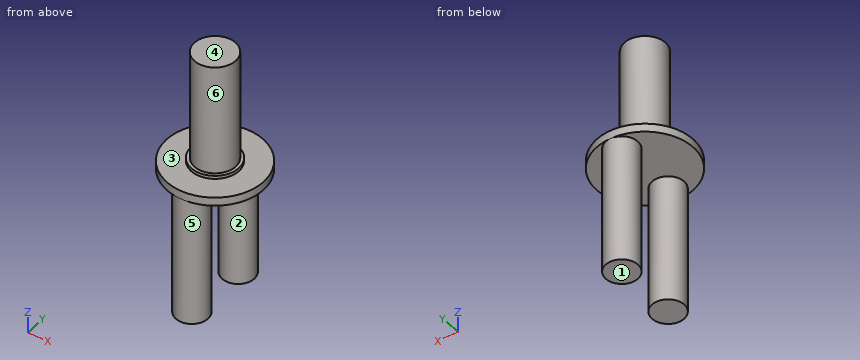
```python
from build123d import *

# Parameters (mm, degrees)
SKETCH1_R             = 1.5875
BOSS_EXTRUDE1_DEPTH   = 12.7
BOSS_EXTRUDE1_2_DEPTH = 12.7
SKETCH2_R             = 2.032
BOSS_EXTRUDE2_DEPTH   = 12.065
SKETCH3_R             = 4.7625
BOSS_EXTRUDE3_DEPTH   = 0.8255
SKETCH4_R             = 2.3495
BOSS_EXTRUDE4_DEPTH   = 0.3175


with BuildPart() as part:
    # Sketch1 → Boss-Extrude1 (new body)
    with BuildSketch(Plane.XY):
        with Locations((0, 12.7)):
            Circle(SKETCH1_R)
    extrude(amount=-BOSS_EXTRUDE1_DEPTH)



with BuildPart() as body_2:
    # Sketch1 → Boss-Extrude1 2 (new body)
    with BuildSketch(Plane.XY):
        with Locations((0, 19.05)):
            Circle(SKETCH1_R)
    extrude(amount=-BOSS_EXTRUDE1_2_DEPTH)


with BuildPart() as part_1:
    add(part.part)

    add(body_2.part)  # Boss-Extrude2 merges body 2
    # Sketch2 → Boss-Extrude2 (add)
    with BuildSketch(Plane.XY):
        with Locations(Location((0, 15.875, 0), (0, 0, 115.050153991))):
            Circle(SKETCH2_R)
    extrude(amount=BOSS_EXTRUDE2_DEPTH)

    # Sketch3 → Boss-Extrude3 (add)
    with BuildSketch(Plane.XY):
        with Locations(Location((0, 15.875, 0), (0, 0, 270))):
            Circle(SKETCH3_R)
    extrude(amount=BOSS_EXTRUDE3_DEPTH)

    # Sketch4 → Boss-Extrude4 (add)
    with BuildSketch(Plane.XY.offset(0.8255)):
        with Locations((0, 15.875)):
            Circle(SKETCH4_R)
    extrude(amount=BOSS_EXTRUDE4_DEPTH)


solid = part_1.part
```
CAD build for the part. Positions are in the model's coordinates, mm. Face numbers are marked on the shaded views. A direction names the side the tool comes from. Coordinates: 2 decimals unless noted, no trailing zeros. Write each loop counter-clockwise with the first axis right and the second up, starting at its lowest first coordinate (ties: lowest second). Pieces come first, ordered by that corner, then holes. Notation, with made-up numbers: (-33, -18.75) -> (11, -18.75) arc R27 ccw to (11, 13.25) -> close; hole circle Ø9 at (88, 42.5). An arc over 180 degrees is marked (long way). Return JSON: item names as keys, results as strings. Group by question number.
Q1. Flat gauge pins, fed straight in: pin 1 (2 mm diameter, centred on y = 12.5, z = -9.5, fed in from +X); pin 2 (5 mm diameter, centred on y = 18, z = -8.5, fed in from -X). Where does each tip first touch, or does it go through?
Q2. Cut at D-D, the plane y = 19.05. Give the cut face in (x, z).
Q3. Pull direction Y, two halves, no side cores. Call the marked faces 4, 5 and 6: released by +Y, released by -Y, zero draft, split by the parting line, or undercut.
Q4. Drill centre lines: line 1 (Z direction, x = 1, y = 12.5); line 2 (Z direction, x = 2.5, y = 15.5); line 3 (Y direction, x = 1.25, z = -6). Where is each one in solid material? Low to high.
Q5. Which spindle directions (+Z, -Z, +X, -X, +Y, -Y) get a long thin tool onto all of the face, cutting with end or side? Do the marked faces 1, 2 and 3. Say none if no direction does.
Returned:
{
 "1": {"pin 1": "stops at x = 1.59", "pin 2": "stops at x = -1.59"},
 "2": {"outline": "(-3.55, 0) -> (-1.59, 0) -> (-1.59, -12.7) -> (1.59, -12.7) -> (1.59, 0) -> (3.55, 0) -> (3.55, 0.83) -> (-3.55, 0.83) -> close"},
 "3": {"face 4": "zero draft", "face 5": "undercut", "face 6": "split by the parting line"},
 "4": {"line 1": "z = -12.7 to 0.83", "line 2": "z = 0 to 0.83", "line 3": "y = 11.72 to 13.68, 18.07 to 20.03"},
 "5": {"face 1": "-Z, +X, -X, +Y, -Y", "face 2": "-Z", "face 3": "+Z"}
}
